Design review of the part built by this model. Coordinates are the model's own, in mm. Face numbers are marked on the shaded views. A direction names the side the tool comes from. Round coordinates to 2 decimals unless told otherwise and drop trailing zeros. Order: outer loops, then holes, each group sorted by start corner. A loop starts at its lowest first (then second) coordinate and runs counter-clockwise, first axis right, second up. Notation, with made-up numbers: (72, -2) - (102, -2) arc R5 cw to (102, 3) - close; hole circle Ø5 at (14, -14). An arc over 180 degrees is marked (long way). Use CSV: the item, a comma, the result in double quotes.
Autodesk Inventor part; units mm, degrees
ref_plane "YZ Plane" through (0, 0, 0) normal (1, 0, 0) x (0, 1, 0)
ref_plane "XZ Plane" through (0, 0, 0) normal (0, 1, 0) x (-1, 0, 0)
ref_plane "XY Plane" through (0, 0, 0) normal (0, 0, 1) x (1, 0, 0)
sketch "Sketch1" plane through (0, 0, 0) normal (0, 1, 0) x (-1, 0, 0)
  line L0 (0, 0) -> (0, -34)
  line L1 (0, -34) -> (11, -45)
  line L2 (11, -45) -> (15, -45)
  line L3 (15, -45) -> (15, -33)
  line L4 (6.7118, 0) -> (0, 0)
  line L5 (15, -33) -> (11, -33)
  line L6 (11, -33) -> (11, -6)
  line L7 (11, -6) -> (25.4, -6)
  line L8 (25.4, -6) -> (25.4, 0)
  line L9 (25.4, 0) -> (6.7118, 0)
  dimension "d0" = 135
  dimension "d1" = 15
  dimension "d2" = 4
  dimension "d13" = 4
  dimension "d14" = 25.4
  dimension "d15" = 6
  dimension "d16" = 12
  dimension "d17" = 45
extrude "Extrusion1" add sketch "Sketch1" along normal mid plane 15
sketch "Sketch2" plane through (-15, -7.5, 0) normal (-1, 0, 0) x (0, 0, 1)
  line L0 (-45, 0) -> (-45, 15)
  circle A0 centre (-39, 7.5) radius 4.0005
  point P0 (0, 7.5)
  point P1 (-45, 7.5)
  dimension "d6" = 6
  dimension "d7" = 8.001
extrude "Extrusion2" cut sketch "Sketch2" against normal through all
sketch "Sketch3" plane through (-11, 7.5, -45) normal (0, 0, -1) x (-1, 0, 0)
  line L0 (4, -15) -> (4, 0)
  line L1 (4, -15) -> (0, -15)
  circle A0 centre (2, -7.5) radius 0.6
  point P0 (-11, -7.5)
  point P1 (2, -15)
  point P2 (4, -7.5)
  dimension "d10" = 1.2
extrude "Extrusion3" cut sketch "Sketch3" against normal up to next
properties part number "focus mount"
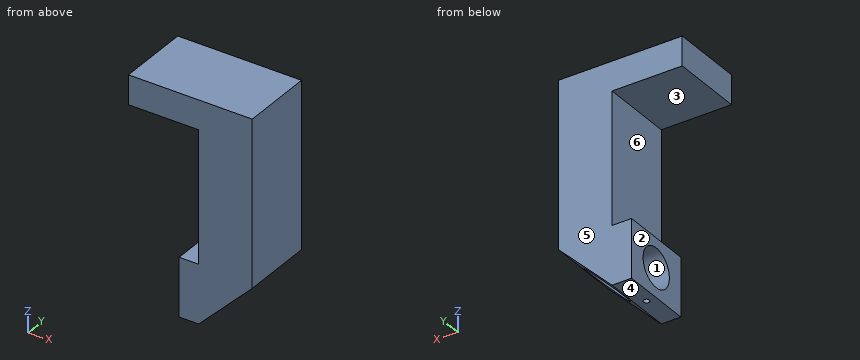
1) We need section B-B (x = -11.5). Give the boundary of the cut face in (y, z), then the cut area to 3 significant figures.
Data:
outline,"(-7.5, -45) - (7.5, -45) - (7.5, -33) - (-7.5, -33) - close; (-7.5, -6) - (7.5, -6) - (7.5, 0) - (-7.5, 0) - close; hole circle Ø8 at (0, -39)"
area,"220 mm2"
2) We need section D-D (y = -2.25). Give the boundary of the cut face in (x, z).
Data:
outline,"(-25.4, -6) - (-11, -6) - (-11, -33) - (-15, -33) - (-15, -35.69) - (-1.69, -35.69) - (0, -34) - (0, 0) - (-25.4, 0) - close; (-15, -45) - (-11, -45) - (-8.31, -42.31) - (-15, -42.31) - close"
3) To check wall thickness, follow L1, parallel to Z at x = -11.75, y = 0; L2, parallel to Y at x = -13, z = -44.25; L3, parallel to Z at x = -13.25, y = 6. State the ranges of each line that lie inside material, in increasing order. Write a range as from..to.
Data:
L1,"z = -45..-43, -35..-33, -6..0"
L2,"y = -7.5..-0.6, 0.6..7.5"
L3,"z = -45..-33, -6..0"
4) The part is to be moulded in two halves that separate along Z. For the marked faces 3, 4, 5 and 6, say which applies: +Z half, -Z half, draft (parallel to the pull), parting line (faces both ways), or undercut.
Data:
face 3,"undercut"
face 4,"-Z half"
face 5,"draft"
face 6,"undercut"
5) Insertion check: pin 1 Ø4.5 at (x, y) = (-16.5, 1.5) entering from -Z; pin 2 Ø8 at (y, z) = (1, -40) entering from -X; pin 3 Ø7.5 at (y, z) = (2, -17) entering from -X. Each pin has a flat end and moves straight along its axis. Give the tip position at first contact, or say it passes through.
Data:
pin 1,"stops at z = -45"
pin 2,"stops at x = -15"
pin 3,"stops at x = -11"
6) We need section C-C (y = 4.5). Give the boundary of the cut face in (x, z).
Data:
outline,"(-25.4, -6) - (-11, -6) - (-11, -33) - (-15, -33) - (-15, -45) - (-11, -45) - (0, -34) - (0, 0) - (-25.4, 0) - close"
7) For the marked faces 1 and 2, list the 3-axis set-ups (+Z, -Z, +X, -X, +Y, -Y) from which the entire face can be reached by the end or side of a thin tool; tool diameter is ignored.
Data:
face 1,"+X, -X"
face 2,"-Z, -X, +Y, -Y"
8) We need section A-A (z = -39). Give the boundary of the cut face in (x, y).
Data:
outline,"(-15, -7.5) - (-5, -7.5) - (-5, -4) - (-15, -4) - close; (-15, 4) - (-5, 4) - (-5, 7.5) - (-15, 7.5) - close"
